```python
from build123d import *

# Parameters (mm, degrees)
SKETCH5_W           = 200
SKETCH5_H           = 200
BOSS_EXTRUDE2_DEPTH = 200
SHELL2_T            = -20
SKETCH6_R           = 30
CUT_EXTRUDE2_DEPTH  = 51.6


with BuildPart() as part:
    # Sketch5 → Boss-Extrude2 (new body)
    with BuildSketch(Plane.XY):
        Rectangle(SKETCH5_W, SKETCH5_H)
    extrude(amount=BOSS_EXTRUDE2_DEPTH)

    # Shell2
    shell2_openings = [part.faces().sort_by_distance(p)[0] for p in [
        (0, 0, 0),
    ]]
    offset(amount=SHELL2_T, openings=shell2_openings, kind=Kind.INTERSECTION)

    # Sketch6 → Cut-Extrude2 (cut)
    with BuildSketch(Plane.XY.offset(200)):
        Circle(SKETCH6_R)
    extrude(amount=-CUT_EXTRUDE2_DEPTH, mode=Mode.SUBTRACT)


solid = part.part
```
Design review of the part built by this model. Coordinates are the model's own, in mm. A direction names the side the tool comes from. Round coordinates to 2 decimals unless told otherwise and drop trailing zeros. Write each loop counter-clockwise with the first axis right and the second up, starting at its lowest first coordinate (ties: lowest second). Pieces come first, ordered by that corner, then holes.
Item 1: We need section A-A on x = 0. Write out the cut boundary in (y, z).
Item 2: Clearance check with a flat-ended pin moving along its axis: pin 1 Ø8 at (x, y) = (0.5, 64) entering from -Z. State where the tip first meets the part, or that it passes through.
Item 3: For probe 1 along Y at (x, z) = (16.5, 10.5); probe 2 along Y at (x, z) = (0, 189.5), list the stretches that pass through material, from the lowest coordinate up.
Item 4: We need section B-B on z = 30. Write out the cut boundary in (x, y).
Item 5: For faces 5 (the flat face through (-1, 100, 99)), 6 (the flat face through (-80, -1, 89)), list the 3-axis set-ups (+Z, -Z, +X, -X, +Y, -Y) from which the entire face can be reached by the end or side of a thin tool; tool diameter is ignored.
Item 6: The part is to be moulded in two halves that separate along X. For faces 1 (the flat face through (100, -1, 99)), 2 (the flat face through (-100, -1, 99)), 3 (the cylindrical face through (-29.97, 1.32, 190.14)), 4 (the flat face through (-90, 1, 0)), say which applies: +X half, -X half, draft (parallel to the pull), parting line (faces both ways), or undercut.
Item 7: We need section D-D on y = -73. Write out the cut boundary in (x, z).
Returned:
1. outline: (-100, 0) - (-80, 0) - (-80, 180) - (-30, 180) - (-30, 200) - (-100, 200) - close; (30, 180) - (80, 180) - (80, 0) - (100, 0) - (100, 200) - (30, 200) - close
2. pin 1: stops at z = 180
3. probe 1: y = -100 to -80, 80 to 100
3. probe 2: y = -100 to -30, 30 to 100
4. outline: (-100, -100) - (100, -100) - (100, 100) - (-100, 100) - close; hole (-80, -80) - (80, -80) - (80, 80) - (-80, 80) - close
5. face 5: +Z, -Z, +X, -X, +Y
5. face 6: -Z
6. face 1: +X half
6. face 2: -X half
6. face 3: undercut
6. face 4: draft
7. outline: (-100, 0) - (-80, 0) - (-80, 180) - (80, 180) - (80, 0) - (100, 0) - (100, 200) - (-100, 200) - close
